from build123d import *

# Parameters (mm, degrees)
SKETCH2_W               = 21.1
SKETCH2_H               = 50.65
SKETCH2_R               = 5.475
BOSS_EXTRUDE1_DEPTH     = 7.5
SKETCH3_W               = 3.15
SKETCH3_H               = 10.25
CUT_EXTRUDE1_DEPTH      = 53.277863384
SKETCH4_W               = 11.1
SKETCH4_H               = 21
CUT_EXTRUDE2_DEPTH      = 13
FILLET1_R               = 0.5
CUT_EXTRUDE3_DEPTH      = 53.277863384
CUT_EXTRUDE3_DEPTH_BACK = 24
SKETCH6_W               = 10
SKETCH6_H               = 3
CUT_EXTRUDE4_START      = -50.65
SKETCH6_2_W             = 10
SKETCH6_2_H             = 3
CUT_EXTRUDE4_DEPTH      = 24
SKETCH7_W               = 11.1
SKETCH7_H               = 5
CUT_EXTRUDE5_DEPTH      = 1


with BuildPart() as part:
    # Sketch2 → Boss-Extrude1 (new, symmetric)
    with BuildSketch(Plane.XY):
        with Locations((0, 6.8)):
            Rectangle(SKETCH2_W, SKETCH2_H)
        Circle(SKETCH2_R, mode=Mode.SUBTRACT)
        with Locations((0, 13.6)):
            Circle(SKETCH2_R, mode=Mode.SUBTRACT)
    extrude(amount=BOSS_EXTRUDE1_DEPTH, both=True)

    # Sketch3 → Cut-Extrude1 (cut, symmetric)
    with BuildSketch(Plane(origin=(0, 32.125, 0), x_dir=(1, 0, 0), z_dir=(0, 1, 0))):
        with Locations((-8.975, 0)):
            Rectangle(SKETCH3_W, SKETCH3_H)
    cut_extrude1 = extrude(amount=CUT_EXTRUDE1_DEPTH, both=True, mode=Mode.SUBTRACT)

    # Mirror1: Cut-Extrude1 across plane
    add(cut_extrude1.mirror(Plane(origin=(0, 0, 0), x_dir=(0, 0, 1), z_dir=(1, 0, 0))), mode=Mode.SUBTRACT)

    # Sketch4 → Cut-Extrude2 (cut)
    with BuildSketch(Plane(origin=(0, 0, -7.5), x_dir=(-1, 0, 0), z_dir=(0, 0, -1))):
        with Locations((0, -5.025)):
            Rectangle(SKETCH4_W, SKETCH4_H)
        with Locations((0, 18.625)):
            Rectangle(SKETCH4_W, SKETCH4_H)
    extrude(amount=-CUT_EXTRUDE2_DEPTH, mode=Mode.SUBTRACT)

    # Fillet1
    fillet1_edges = [part.edges().sort_by_distance(p)[0] for p in [
        (-7.4, 6.8, -5.125),
        (-7.4, 6.8, 5.125),
        (7.4, 6.8, 5.125),
        (7.4, 6.8, -5.125),
    ]]
    fillet(fillet1_edges, radius=FILLET1_R)

    # Sketch6 → Cut-Extrude3 (cut, two sides: drawn at the far end of the back side and taken through both)
    with BuildSketch(Plane(origin=(0, 32.125, 0), x_dir=(1, 0, 0), z_dir=(0, 1, 0)).offset(-CUT_EXTRUDE3_DEPTH_BACK)):
        with Locations((0, 4.5)):
            Rectangle(SKETCH6_W, SKETCH6_H)
    extrude(amount=CUT_EXTRUDE3_DEPTH + CUT_EXTRUDE3_DEPTH_BACK, mode=Mode.SUBTRACT)

    # Sketch6<2> → Cut-Extrude4 (cut)
    with BuildSketch(Plane(origin=(0, 32.125, 0), x_dir=(1, 0, 0), z_dir=(0, 1, 0)).offset(CUT_EXTRUDE4_START)):
        with Locations((0, 4.5)):
            Rectangle(SKETCH6_2_W, SKETCH6_2_H)
    extrude(amount=CUT_EXTRUDE4_DEPTH, mode=Mode.SUBTRACT)

    # Sketch7 → Cut-Extrude5 (cut)
    with BuildSketch(Plane(origin=(0, 0, 5.5), x_dir=(-1, 0, 0), z_dir=(0, 0, -1))):
        with Locations((0, 26.625)):
            Rectangle(SKETCH7_W, SKETCH7_H)
        with Locations((0, -13.025)):
            Rectangle(SKETCH7_W, SKETCH7_H)
    extrude(amount=-CUT_EXTRUDE5_DEPTH, mode=Mode.SUBTRACT)


solid = part.part
Part model, mm, in its own coordinate system. A direction names the side the tool comes from. Round coordinates to 2 decimals unless told otherwise and drop trailing zeros. Loops run counter-clockwise (first coordinate to the right, second up) from the corner with the lowest first, then second, coordinate; pieces in that order, holes last. Notation, with made-up numbers: (-31.75, -6) - (-6.75, -6) arc R11 cw to (-6.75, 2) - close; hole circle Ø2 at (22.5, -31.75). An arc over 180 degrees is marked (long way). Answer as a JSON object with one key per item and string values.
Item 1: Band-saw the part on A-A on x = -8.75. List the corners of the cut face in (y, z) (3 decimals).
Output:
{"outline": "(-18.525, -7.5) - (32.125, -7.5) - (32.125, -5.125) - (-18.525, -5.125) - close; (-18.525, 5.125) - (32.125, 5.125) - (32.125, 7.5) - (-18.525, 7.5) - close"}
Item 2: Wall check: L1, parallel to Y at x = 0, z = 6.2 (3 decimals); L2, parallel to Y at x = -2, z = -0.5 (3 decimals); L3, parallel to X at y = 17.5, z = -3.75. Give the ranges that are in metal, low to high.
Output:
{"L1": "-18.525 to -15.525, -10.525 to -5.475, 5.475 to 8.125, 19.075 to 24.125, 29.125 to 32.125", "L2": "-18.525 to -15.525, 5.475 to 8.125, 29.125 to 32.125", "L3": "-7.4 to -5.55, 5.55 to 7.4"}
Item 3: Band-saw the part on C-C on z = 2. List the corners of the cut face in (x, y) (3 decimals).
Output:
{"outline": "(-7.4, -18.525) - (7.4, -18.525) - (7.4, 32.125) - (-7.4, 32.125) - close; hole (-5.55, -15.525) - (5.55, -15.525) - (5.55, 5.475) - (-5.55, 5.475) - close; hole (-5.55, 8.125) - (5.55, 8.125) - (5.55, 29.125) - (-5.55, 29.125) - close"}
Item 4: Tool access for faces 1 (the face through (0, 20, 5.5)), 2 (the face through (-9, 7, -5.125)), 3 (the face through (0, -17, -6)), 4 (the face through (0, 31, -3)): list every direction of +Z, -Z, +X, -X, +Y, -Y with a clear straight run to the whole face (end or side of a thin tool).
Output:
{"face 1": "-Z", "face 2": "-X, +Y, -Y", "face 3": "-Y", "face 4": "+Y"}
Item 5: Pin check, flat tips, straight feed: pin 1 (2.5 mm diameter, centred on x = -1.5, y = -12.5, fed in from -Z); pin 2 (4.5 mm diameter, centred on y = 4, z = 1, fed in from -X); pin 3 (6 mm diameter, centred on y = 0, z = -1.5, fed in from +X). Stop position of each tip, or through.
Output:
{"pin 1": "z = 6.5", "pin 2": "x = -7.4", "pin 3": "x = 7.4"}
Item 6: Band-saw the part on B-B on y = 0. List the corners of the cut face in (x, z) (3 decimals), plus the area to 3 significant figures.
Output:
{"outline": "(-10.55, -7.5) - (-5.55, -7.5) - (-5.55, 5.5) - (-5.475, 5.5) - (-5.475, 7.5) - (-10.55, 7.5) - (-10.55, 5.125) - (-7.9, 5.125) arc R0.5 cw to (-7.4, 4.625) - (-7.4, -4.625) arc R0.5 cw to (-7.9, -5.125) - (-10.55, -5.125) - close; (5.475, 5.5) - (5.55, 5.5) - (5.55, -7.5) - (10.55, -7.5) - (10.55, -5.125) - (7.9, -5.125) arc R0.5 cw to (7.4, -4.625) - (7.4, 4.625) arc R0.5 cw to (7.9, 5.125) - (10.55, 5.125) - (10.55, 7.5) - (5.475, 7.5) - close", "area": "85.9 mm2"}
Item 7: Band-saw the part on D-D on x = -4.25. State how many separate pieces and enclosed holes the cut face has, plus the area to 3 significant figures.
Output:
{"separate pieces": "5", "enclosed holes": "0", "area": "158 mm2"}
Item 8: Pull direction Y, two halves, no side cores. Call faces 5 (the face through (0, 8.125, -1)), 6 (the face through (10.55, 6, 6)), 7 (the face through (0, 32.125, 0)): pulls with the +Y half, pulls with the -Y half, needs draft (parallel to the pull), parting line crosses it, or undercut.
Output:
{"face 5": "undercut", "face 6": "needs draft", "face 7": "pulls with the +Y half"}
